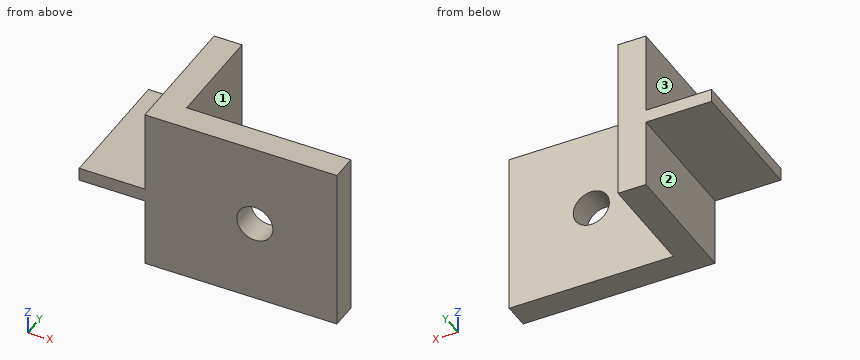
```python
from build123d import *

# Parameters (mm, degrees)
SKETCH_1_W          = 25
SKETCH_1_H          = 25
SKETCH_1_R          = 2.75
EXTRUDE_1_DEPTH     = 4
SKETCH_1_3_W        = 15
SKETCH_1_3_H        = 25
EXTRUDE_2_DEPTH     = 20
SKETCH_2_W          = 10.750885586
SKETCH_2_H          = 25
CUT_EXTRUDE_1_DEPTH = 43
SKETCH_3_W          = 10
SKETCH_3_H          = 2
EXTRUDE_4_DEPTH     = 20


with BuildPart() as part:
    # 草图1 → 凸台-拉伸1 (new body)
    with BuildSketch(Plane(origin=(0, 0, 0), x_dir=(1, 0, 0), z_dir=(0, 1, 0))):
        Rectangle(SKETCH_1_W, SKETCH_1_H)
        with Locations(Location((0, 0, 0), (0, 0, 270))):
            Circle(SKETCH_1_R, mode=Mode.SUBTRACT)
    extrude(amount=EXTRUDE_1_DEPTH)

    # 草图1<3> → 凸台-拉伸2 (add)
    with BuildSketch(Plane(origin=(0, 0, 0), x_dir=(1, 0, 0), z_dir=(0, 1, 0))):
        with Locations((-20, 0)):
            Rectangle(SKETCH_1_3_W, SKETCH_1_3_H)
    extrude(amount=EXTRUDE_2_DEPTH)

    # 草图2 → 切除-拉伸1 (cut)
    with BuildSketch(Plane(origin=(0, 20, 0), x_dir=(1, 0, 0), z_dir=(0, 1, 0))):
        with Locations((-22.124557207, 0)):
            Rectangle(SKETCH_2_W, SKETCH_2_H)
    extrude(amount=-CUT_EXTRUDE_1_DEPTH, mode=Mode.SUBTRACT)

    # 草图3 → 凸台-拉伸4 (add)
    with BuildSketch(Plane(origin=(0, 20, 0), x_dir=(1, 0, 0), z_dir=(0, 1, 0))):
        with Locations((-21.749114414, 1)):
            Rectangle(SKETCH_3_W, SKETCH_3_H)
    extrude(amount=-EXTRUDE_4_DEPTH)


solid = part.part
```
The model under review builds one solid part; all positions refer to its coordinate system, in mm. Face numbers are marked on the shaded views. A direction names the side the tool comes from. Coordinates: 2 decimals unless noted, no trailing zeros. Write each loop counter-clockwise with the first axis right and the second up, starting at its lowest first coordinate (ties: lowest second). Pieces come first, ordered by that corner, then holes.
1) To check wall thickness, follow probe 1 along X at (y, z) = (11.75, 7); probe 2 along Y at (x, z) = (-12, -4.5); probe 3 along X at (y, z) = (2, -1.75). State the ranges of each line that lie inside material, in increasing order.
2) Clearance check with flat-ended pins moving along their axes: pin 1 Ø5 at (y, z) = (13, 3.5) entering from +X; pin 2 Ø2 at (x, z) = (8.5, 7.5) entering from -Y; pin 3 Ø6.5 at (x, z) = (0, 0) entering from +Y; pin 4 Ø10 at (y, z) = (14.5, -9) entering from -X. State where each tip first meets the part, or that it passes through.
3) We need section B-B on x = 0. State the section outline as (y, z) points.
4) Machinability: for the marked faces 1, 2 and 3, which of the approach directions +Z, -Z, +X, -X, +Y, -Y give a long, thin tool a straight path to every point of the face, cutting with its end or side? Answer none if there is none.
5) We need section A-A on y = 3.5. State the section outline as (x, z) points, then the cut area to 3 significant figures.
6) We need section D-D on y = 15. State the section outline as (x, z) points, then the cut area to 3 significant figures.
7) We need section C-C on z = 0.5. State the section outline as (x, y) points, then the cut area to 3 significant figures.
Answer list:
1. probe 1: x = -16.75 to -12.5
1. probe 2: y = 0 to 4
1. probe 3: x = -26.75 to -2.12, 2.12 to 12.5
2. pin 1: stops at x = -12.5
2. pin 2: stops at y = 0
2. pin 3: stops at y = 4
2. pin 4: stops at x = -16.75
3. outline: (0, -12.5) - (4, -12.5) - (4, -2.75) - (0, -2.75) - close; (0, 2.75) - (4, 2.75) - (4, 12.5) - (0, 12.5) - close
4. face 1: +Z, -Z, +X, +Y
4. face 2: -Z, -X, +Y, -Y
4. face 3: +Z, -X, +Y, -Y
5. outline: (-26.75, -2) - (-16.75, -2) - (-16.75, -12.5) - (12.5, -12.5) - (12.5, 12.5) - (-16.75, 12.5) - (-16.75, 0) - (-26.75, 0) - close; hole circle Ø5.5 at (0, 0)
5. area: 727 mm2
6. outline: (-26.75, -2) - (-16.75, -2) - (-16.75, -12.5) - (-12.5, -12.5) - (-12.5, 12.5) - (-16.75, 12.5) - (-16.75, 0) - (-26.75, 0) - close
6. area: 126 mm2
7. outline: (-16.75, 0) - (-2.7, 0) - (-2.7, 4) - (-12.5, 4) - (-12.5, 20) - (-16.75, 20) - close; (2.7, 0) - (12.5, 0) - (12.5, 4) - (2.7, 4) - close
7. area: 163 mm2
